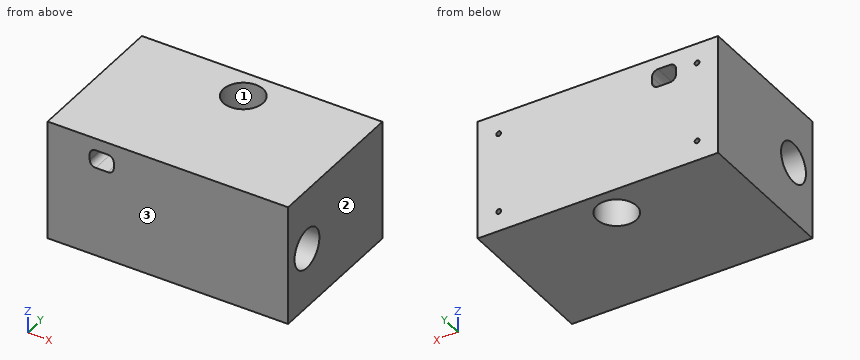
from build123d import *

# Parameters (mm, degrees)
SKETCH1_W           = 50.8
SKETCH1_H           = 31.75
BOSS_EXTRUDE1_DEPTH = 25.4
SKETCH4_R           = 4.191
CUT_EXTRUDE1_DEPTH  = 152.4
SKETCH5_R           = 4.191
CUT_EXTRUDE2_DEPTH  = 25.4
SKETCH7_R           = 0.508
CUT_EXTRUDE3_DEPTH  = 7.62
SKETCH9_W           = 5.08
SKETCH9_H           = 3.81
CUT_EXTRUDE5_DEPTH  = 152.4
FILLET1_R           = 1.27


with BuildPart() as part:
    # Sketch1 → Boss-Extrude1 (new body)
    with BuildSketch(Plane.XY):
        Rectangle(SKETCH1_W, SKETCH1_H)
    extrude(amount=BOSS_EXTRUDE1_DEPTH)

    # Sketch4 → Cut-Extrude1 (cut)
    with BuildSketch(Plane.ZY.offset(25.4)):
        with Locations((12.7, -9.525)):
            Circle(SKETCH4_R)
    extrude(amount=-CUT_EXTRUDE1_DEPTH, mode=Mode.SUBTRACT)

    # Sketch5 → Cut-Extrude2 (cut)
    with BuildSketch(Plane.XY.offset(25.4)):
        with Locations((0, 9.525)):
            Circle(SKETCH5_R)
    extrude(amount=-CUT_EXTRUDE2_DEPTH, mode=Mode.SUBTRACT)

    # Sketch7 → Cut-Extrude3 (cut)
    with BuildSketch(Plane(origin=(0, 15.875, 0), x_dir=(1, 0, 0), z_dir=(0, 1, 0))):
        with Locations((-20.955, -4.2291)):
            Circle(SKETCH7_R)
        with Locations((-20.955, -21.1709)):
            Circle(SKETCH7_R)
        with Locations((20.955, -4.2291)):
            Circle(SKETCH7_R)
        with Locations((20.955, -21.1709)):
            Circle(SKETCH7_R)
    extrude(amount=-CUT_EXTRUDE3_DEPTH, mode=Mode.SUBTRACT)

    # Sketch9 → Cut-Extrude5 (cut)
    with BuildSketch(Plane(origin=(0, 15.875, 0), x_dir=(1, 0, 0), z_dir=(0, 1, 0))):
        with Locations((-13.97, -20.955)):
            Rectangle(SKETCH9_W, SKETCH9_H)
    extrude(amount=-CUT_EXTRUDE5_DEPTH, mode=Mode.SUBTRACT)

    # Fillet1
    fillet1_edges = [part.edges().sort_by_distance(p)[0] for p in [
        (-16.51, 0, 22.86),
        (-16.51, 0, 19.05),
        (-11.43, 0, 19.05),
        (-11.43, 0, 22.86),
    ]]
    fillet(fillet1_edges, radius=FILLET1_R)


solid = part.part
Can you work these out from the model? Positions are in its coordinate system, mm. Face numbers are marked on the shaded views. Coordinates: 2 decimals unless noted, no trailing zeros. Write each loop counter-clockwise with the first axis right and the second up, starting at its lowest first coordinate (ties: lowest second). Pieces come first, ordered by that corner, then holes. Notation, with made-up numbers: (34.25, 38) -> (74.25, 38) arc R15 cw to (74.25, 43) -> close; hole circle Ø5 at (21, 38.5). An arc over 180 degrees is marked (long way). Write each question's results on one line, items separated by ' | '. Start each with the question number.
Item 1: If we section it at D-D, the plane y = -11.5: Write out the boundary of the cut face in (x, z), and give its area (3 significant figures).
Item 2: Thinking about a two-plate mould opening in X: for the marked faces 1, 2 and 3, which applies, released by +X, released by -X, zero draft, split by the parting line, or undercut?
Item 3: I'm going to push flat-ended pins straight in: P1, Ø0.6, axis at x = -20.96, z = 21.17, coming from the +Y side (3 decimals); P2, Ø6.5, axis at y = -9.525, z = 12.7, coming from the +X side. Where does each tip first touch, or does it pass through?
Item 4: Please list where these lines run through material, in increasing order: probe 1 along Y at (x, z) = (1, 15) (1 decimal); probe 2 along Y at (x, z) = (0, 11.75) (3 decimals); probe 3 along Y at (x, z) = (-23, 12.5) (3 decimals).
Item 5: If we section it at B-B, the plane x = 0: Write out the boundary of the cut face in (y, z) (3 decimals).
Item 6: If we section it at C-C, the plane y = 12.5: Write out the boundary of the cut face in (x, z) (3 decimals).
Item 7: If we section it at A-A, the plane z = 12: Write out the boundary of the cut face in (x, y) (3 decimals).
Answer block:
1) outline: (-25.4, 0) -> (25.4, 0) -> (25.4, 9) -> (-25.4, 9) -> close; (-25.4, 16.4) -> (25.4, 16.4) -> (25.4, 25.4) -> (-25.4, 25.4) -> close; hole (-16.51, 20.32) arc R1.27 ccw to (-15.24, 19.05) -> (-12.7, 19.05) arc R1.27 ccw to (-11.43, 20.32) -> (-11.43, 21.59) arc R1.27 ccw to (-12.7, 22.86) -> (-15.24, 22.86) arc R1.27 ccw to (-16.51, 21.59) -> close | area: 897 mm²
2) face 1: undercut | face 2: released by +X | face 3: zero draft
3) P1: y = 8.255 | P2: through
4) probe 1: -15.9 to -13, -6 to 5.5, 13.6 to 15.9 | probe 2: -15.875 to -13.607, -5.443 to 5.334, 13.716 to 15.875 | probe 3: -15.875 to -13.711, -5.339 to 15.875
5) outline: (-15.875, 0) -> (5.334, 0) -> (5.334, 25.4) -> (-15.875, 25.4) -> close; (13.716, 0) -> (15.875, 0) -> (15.875, 25.4) -> (13.716, 25.4) -> close; hole circle Ø8.382 at (-9.525, 12.7)
6) outline: (-25.4, 0) -> (-2.952, 0) -> (-2.952, 25.4) -> (-25.4, 25.4) -> close; (2.952, 0) -> (25.4, 0) -> (25.4, 25.4) -> (2.952, 25.4) -> close; hole circle Ø1.016 at (-20.955, 4.229); hole circle Ø1.016 at (-20.955, 21.171); hole (-16.51, 20.32) arc R1.27 ccw to (-15.24, 19.05) -> (-12.7, 19.05) arc R1.27 ccw to (-11.43, 20.32) -> (-11.43, 21.59) arc R1.27 ccw to (-12.7, 22.86) -> (-15.24, 22.86) arc R1.27 ccw to (-16.51, 21.59) -> close; hole circle Ø1.016 at (20.955, 4.229); hole circle Ø1.016 at (20.955, 21.171)
7) outline: (-25.4, -15.875) -> (25.4, -15.875) -> (25.4, -13.657) -> (-25.4, -13.657) -> close; (-25.4, -5.393) -> (25.4, -5.393) -> (25.4, 15.875) -> (-25.4, 15.875) -> close; hole circle Ø8.382 at (0, 9.525)
